Input: part model. Units: mm. Frame: model coordinates. Round coordinates to 2 decimals unless told otherwise and drop trailing zeros. Answer as a JSON object with one key per item and string values.
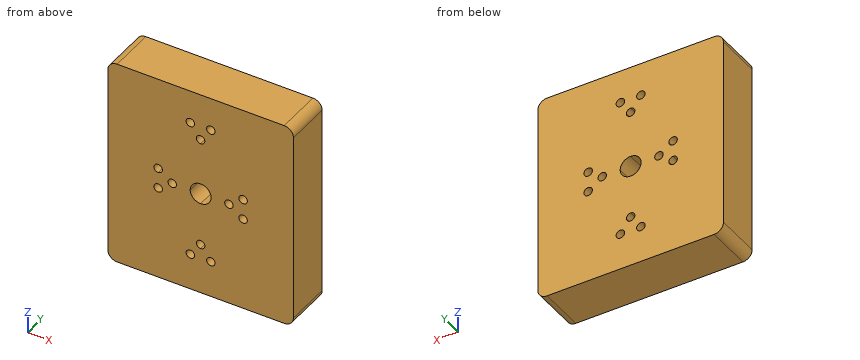
```python
from build123d import *

# Parameters (mm, degrees)
F0_W     = 101.6
F0_H     = 114.3
F1_DEPTH = 25.4
F2_R     = 2.3241
F3_DEPTH = 25.401
F4_R     = 5.08


with BuildPart() as f1:
    # F0 (on Front) → F1 (new body)
    with BuildSketch(Plane.XZ):
        Rectangle(F0_W, F0_H)
    extrude(amount=F1_DEPTH)

    # F2 (on face) → F3 (cut, through all)
    with BuildSketch(Plane.XZ.offset(25.4)):
        with BuildLine():
            ThreePointArc((0, -5.715), (4.041115, -4.041115), (5.715, 0))
            ThreePointArc((5.715, 0), (4.041115, 4.041115), (0, 5.715))
            ThreePointArc((0, 5.715), (-4.041115, 4.041115), (-5.715, 0))
            ThreePointArc((-5.715, 0), (-4.041115, -4.041115), (0, -5.715))
        make_face()
        with BuildLine():
            ThreePointArc((2.3241, -29.3243), (1.643387, -27.680913), (0, -27.0002))
            Line((0, -27.0002), (0, -31.6484))
            ThreePointArc((0, -31.6484), (1.643387, -30.967687), (2.3241, -29.3243))
        make_face()
        with BuildLine():
            Line((0, -31.6484), (0, -27.0002))
            ThreePointArc((0, -27.0002), (-2.3241, -29.3243), (0, -31.6484))
        make_face()
        with BuildLine():
            ThreePointArc((-20.9169, -5.6261), (-21.597613, -3.982713), (-23.241, -3.302))
            ThreePointArc((-23.241, -3.302), (-24.884387, -7.269487), (-20.9169, -5.6261))
        make_face()
        with BuildLine():
            ThreePointArc((-20.9169, 5.6261), (-24.884387, 7.269487), (-23.241, 3.302))
            ThreePointArc((-23.241, 3.302), (-21.597613, 3.982713), (-20.9169, 5.6261))
        make_face()
        with BuildLine():
            ThreePointArc((-17.8308, 0), (-15.5067, -2.3241), (-13.1826, 0))
            ThreePointArc((-13.1826, 0), (-15.5067, 2.3241), (-17.8308, 0))
        make_face()
        with Locations((-5.6134, 38.9636)):
            Circle(F2_R)
        with BuildLine():
            ThreePointArc((7.9375, 38.9636), (5.6134, 41.2877), (3.2893, 38.9636))
            ThreePointArc((3.2893, 38.9636), (5.6134, 36.6395), (7.9375, 38.9636))
        make_face()
        with BuildLine():
            ThreePointArc((0, 33.5534), (-2.3241, 31.2293), (0, 28.9052))
            Line((0, 28.9052), (0, 33.5534))
        make_face()
        with BuildLine():
            Line((0, 33.5534), (0, 28.9052))
            ThreePointArc((0, 28.9052), (1.643387, 29.585913), (2.3241, 31.2293))
            ThreePointArc((2.3241, 31.2293), (1.643387, 32.872687), (0, 33.5534))
        make_face()
        with Locations((-5.6134, -37.0586)):
            Circle(F2_R)
        with Locations((5.6134, -37.0586)):
            Circle(F2_R)
        with Locations((15.5067, 0)):
            Circle(F2_R)
        with Locations((23.241, -5.6261)):
            Circle(F2_R)
        with Locations((23.241, 5.6261)):
            Circle(F2_R)
    extrude(amount=-F3_DEPTH, mode=Mode.SUBTRACT)

    # F4
    f4_edges = [f1.edges().sort_by_distance(p)[0] for p in [
        (-50.8, -12.7, -57.15),
        (50.8, -12.7, -57.15),
        (-50.8, -12.7, 57.15),
        (50.8, -12.7, 57.15),
    ]]
    fillet(f4_edges, radius=F4_R)


solid = f1.part
```
1) Ray query, probe 1 along X at (y, z) = (-7.25, -6); probe 2 along X at (y, z) = (-8, -5); probe 3 along X at (y, z) = (-8, -1). Return the intervals inside material, ascending.
Output:
{"probe 1": "x = -50.8 to -25.53, -20.95 to 20.95, 25.53 to 50.8", "probe 2": "x = -50.8 to -25.48, -21 to -2.77, 2.77 to 21, 25.48 to 50.8", "probe 3": "x = -50.8 to -17.6, -13.41 to -5.63, 5.63 to 13.41, 17.6 to 50.8"}
2) Section A-A, the plane y = -7.25. Count the separate pieces of the cut face and the enclosed holes in it, plus the area to 3 significant figures.
Output:
{"separate pieces": "1", "enclosed holes": "13", "area": "11,300 mm^2"}
3) Contact query for a flat-ended pin moving along its axis: P1, Ø3, axis at x = -5.61, z = 38.96, coming from the -Y side. Output: stop coordinate, or through.
Output:
{"P1": "passes through"}
